from build123d import *

# Parameters (mm, degrees)
SKETCH_1_R          = 5
EXTRUDE_1_DEPTH     = 3
CUT_EXTRUDE_1_DEPTH = 3
FILLET_2_R          = 2


with BuildPart() as part:
    # 草图1 → 凸台-拉伸1 (new body)
    with BuildSketch(Plane(origin=(0, 0, 0), x_dir=(1, 0, 0), z_dir=(0, 1, 0))):
        with BuildLine():
            Line((-1.330576007, 11.926003836), (80, 21))
            Line((80, 21), (240.672524597, 11.98113979))
            ThreePointArc((240.672524597, 11.98113979), (252, 0), (240.672524597, -11.98113979))
            Line((240.672524597, -11.98113979), (80, -21))
            Line((80, -21), (-1.330576007, -11.926003836))
            ThreePointArc((-1.330576007, -11.926003836), (-12, 0), (-1.330576007, 11.926003836))
        make_face()
        with Locations(Location((0, 0, 0), (0, 0, 270))):
            Circle(SKETCH_1_R, mode=Mode.SUBTRACT)
        with Locations(Location((80, 0, 0), (0, 0, 270))):
            Circle(SKETCH_1_R, mode=Mode.SUBTRACT)
        with Locations(Location((240, 0, 0), (0, 0, 270))):
            Circle(SKETCH_1_R, mode=Mode.SUBTRACT)
    extrude(amount=EXTRUDE_1_DEPTH)

    # 圆角1
    # a fillet whose section is not a circle: 40 mm, written as the material it takes off along each edge
    with BuildSketch(Plane(origin=(80, -8.378669722, 21), x_dir=(0.9984283158275346, 0, -0.0560437164523641), z_dir=(0, 1, 0)), Plane(origin=(80, -8.378669722, -21), x_dir=(-0.9938336529777407, 0, 0.1108813339066567), z_dir=(0, 1, 0))) as fillet_1_piece_1:
        with BuildLine():
            add(Edge.make_bspline([(3.351467889, 0), (2.723727072, 0), (2.095986256, 0), (0.700623386, 0.02340826), (-0.686959659, 0.139669261), (-2.06676288, 0.348783001), (-2.685751394, 0.453242334), (-3.304739908, 0.557701667)], knots=[0, 0, 0, 0, 0, 0, 0.5, 0.5, 1, 1, 1, 1, 1, 1], degree=5))
            Line((-3.304739908, 0.557701667), (0, 0))
            Line((0, 0), (3.351467889, 0))
        make_face()
    extrude(amount=19.757339444, mode=Mode.SUBTRACT)

    # 草图2 → 切除-拉伸1 (cut)
    with BuildSketch(Plane.XZ):
        Polygon((8.062257748, 4), (65.387758913, 15.344903932), (71.937742252, 4), align=None)
        Polygon((88.062257748, 4), (107.859425007, 15.429899846), (231.937742252, 4), align=None)
        Polygon((107.859425007, -15.429899846), (231.937742252, -4), (88.062257748, -4), align=None)
        Polygon((65.387758913, -15.344903932), (71.937742252, -4), (8.062257748, -4), align=None)
    extrude(amount=-CUT_EXTRUDE_1_DEPTH, mode=Mode.SUBTRACT)

    # 圆角2
    fillet_2_edges = [part.edges().sort_by_distance(p)[0] for p in [
        (65.387758913, 1.5, -15.344903932),
        (8.062257748, 1.5, -4),
        (71.937742252, 1.5, -4),
        (107.859425007, 1.5, -15.429899846),
        (88.062257748, 1.5, -4),
        (231.937742252, 1.5, -4),
        (231.937742252, 1.5, 4),
        (88.062257748, 1.5, 4),
        (107.859425007, 1.5, 15.429899846),
        (71.937742252, 1.5, 4),
        (8.062257748, 1.5, 4),
        (65.387758913, 1.5, 15.344903932),
    ]]
    fillet(fillet_2_edges, radius=FILLET_2_R)


solid = part.part
Verification items for the finished model (mm, model axes). A direction names the side the tool comes from. Round coordinates to 2 decimals unless told otherwise and drop trailing zeros. Order: outer loops, then holes, each group sorted by start corner. A loop starts at its lowest first (then second) coordinate and runs counter-clockwise, first axis right, second up.
1. Thickness scan on L1, parallel to X at y = 2.45, z = 0.5; L2, parallel to Z at x = 97.5, y = 2.25; L3, parallel to X at y = 0.3, z = 3.5. Record the ranges inside material, lowest first.
Final values:
L1: x = -11.99 to -4.97, 4.97 to 75.03, 84.97 to 235.03, 244.97 to 251.99
L2: z = -20.02 to -9.45, -4 to 4, 9.45 to 20.02
L3: x = -11.48 to -3.57, 3.57 to 76.43, 83.57 to 236.43, 243.57 to 251.48
2. Section check B-B on y = 1.7. State how many separate pieces and enclosed holes the cut face has, then the cut area to 3 significant figures.
Final values:
separate pieces: 1
enclosed holes: 7
area: 6,030 mm2
3. Go/stop test with flat-tipped pins: P1, Ø9, axis at x = 0, z = 0, coming from the +Y side; P2, Ø1.5, axis at x = 56.5, y = 1, coming from the -Z side; P3, Ø1.5, axis at y = 1, z = 6, coming from the -X side; P4, Ø1.5, axis at x = 89.5, y = 1.5, coming from the +Z side. Record where each tip stops, or that it passes through.
Final values:
P1: passes through
P2: stops at z = -18.46
P3: stops at x = -10.79
P4: stops at z = 20.51
4. Release check for a two-part mould opening along X. For faces 3 (the cylindrical face through (252, 1, 0)), 4 (the cylindrical face through (-12, 1, 0)), 5 (the flat face through (147.989, 1.479, -11.733)) record: +X half, -X half, draft (parallel to the pull), parting line (faces both ways), or undercut.
Final values:
face 3: +X half
face 4: -X half
face 5: undercut
5. Access from +Z, -Z, +X, -X, +Y, -Y to the whole of each face (thin tool, end or side, straight path). Record for faces 1 (the flat face through (37.123, 1.479, -16.216)), 2 (the flat face through (100.83, 1.48, 11.37)).
Final values:
face 1: -Z, -X, +Y, -Y
face 2: +Y, -Y
6. Section check A-A on z = 0. Record the cut outline in (x, y), then the cut area to 3 significant figures.
Final values:
outline: (-12, 0) - (-5, 0) - (-5, 3) - (-12, 3) - close; (5, 0) - (75, 0) - (75, 3) - (5, 3) - close; (85, 0) - (235, 0) - (235, 3) - (85, 3) - close; (245, 0) - (252, 0) - (252, 3) - (245, 3) - close
area: 702 mm2
7. Section check C-C on x = 231.5. Record the cut outline in (y, z).
Final values:
outline: (0, -12.5) - (3, -12.5) - (3, 12.5) - (0, 12.5) - close
